Here's how the part is built. I have some questions about the finished solid (model axes, mm). Coordinates: 2 decimals unless noted, no trailing zeros. Write each loop counter-clockwise with the first axis right and the second up, starting at its lowest first coordinate (ties: lowest second). Pieces come first, ordered by that corner, then holes.
(1) Please list where these lines run through material, in increasing order: probe 1 along Y at (x, z) = (-4.5, 50); probe 2 along Z at (x, y) = (0, 70) (3 decimals); probe 3 along Z at (x, y) = (0, -1) (3 decimals).
(2) For pin 1 Ø1.5 at (x, y) = (11, 23.5) entering from +Z; pin 2 Ø2 at (x, y) = (16, -0.5) entering from +Z, each with a flat end and sliding along its axis, tell me the tip position at first contact or that it passes through.
(3) Thinking about a two-plate mould opening in Y: for faces 1 (the cylindrical face through (14.65, -1.07, -28.17)), 2 (the flat face through (0, -76.2, 37)), 3 (the flat face through (31.75, 64, 36)), which applies, released by +Y, released by -Y, zero draft, split by the parting line, or undercut?
(4) Imagine slicing it at D-D, the plane z = 75.5. List the corners of the cut face in (x, y) for me.
(5) Imagine slicing it at A-A, the plane z = 43. List the corners of the cut face in (x, y) for me.
(6) Imagine slicing it at C-C, the plane y = -54.5. List the corners of the cut face in (x, z) for me (3 decimals).
(7) Imagine slicing it at B-B, the plane x = 0. List the corners of the cut face in (y, z) for me (3 decimals).
```python
from build123d import *

# Parameters (mm, degrees)
F0_R     = 31.75
F0_R_2   = 15.875
F1_DEPTH = 76.2
F3_DEPTH = 25.4
F5_R     = 15.875
F6_DEPTH = 152.401


with BuildPart() as f1:
    # F0 (on Front) → F1 (new body, symmetric)
    with BuildSketch(Plane.XZ):
        Circle(F0_R)
        Circle(F0_R_2, mode=Mode.SUBTRACT)
    extrude(amount=F1_DEPTH, both=True)

    # F2 (on face) → F3 (join)
    with BuildSketch(Plane.XZ.offset(76.2)):
        with BuildLine():
            ThreePointArc((31.75, 72.5937485695), (0, 104.3437485695), (-31.75, 72.5937485695))
            Line((-31.75, 72.5937485695), (31.75, 72.5937485695))
        make_face()
        with BuildLine():
            Line((31.75, 72.5937485695), (-31.75, 72.5937485695))
            ThreePointArc((-31.75, 72.5937485695), (0, 40.8437485695), (31.75, 72.5937485695))
        make_face()
        with BuildLine():
            Line((-31.75, 72.5937485695), (-31.75, 0))
            ThreePointArc((-31.75, 0), (0, 31.75), (31.75, 0))
            Line((31.75, 0), (31.75, 72.5937485695))
            ThreePointArc((31.75, 72.5937485695), (0, 40.8437485695), (-31.75, 72.5937485695))
        make_face()
    extrude(amount=-F3_DEPTH)

    # F4: F1 across plane


with BuildPart() as f1_1:
    add(f1.part)
    add(f1.part.mirror(Plane.XZ))

    # F5 (on face) → F6 (cut, through all)
    with BuildSketch(Plane.XZ.offset(76.2)):
        with Locations((0, 72.5937485695)):
            Circle(F5_R)
    extrude(amount=-F6_DEPTH, mode=Mode.SUBTRACT)


solid = f1_1.part
```
Recorded:
1. probe 1: y = -76.2 to -50.8, 50.8 to 76.2
1. probe 2: z = -31.75 to -15.875, 15.875 to 56.719, 88.469 to 104.344
1. probe 3: z = -31.75 to -15.875, 15.875 to 31.75
2. pin 1: stops at z = 30.05
2. pin 2: stops at z = 27.98
3. face 1: undercut
3. face 2: released by -Y
3. face 3: zero draft
4. outline: (-31.62, -76.2) - (-15.61, -76.2) - (-15.61, -50.8) - (-31.62, -50.8) - close; (-31.62, 50.8) - (-15.61, 50.8) - (-15.61, 76.2) - (-31.62, 76.2) - close; (15.61, -76.2) - (31.62, -76.2) - (31.62, -50.8) - (15.61, -50.8) - close; (15.61, 50.8) - (31.62, 50.8) - (31.62, 76.2) - (15.61, 76.2) - close
5. outline: (-31.75, -76.2) - (31.75, -76.2) - (31.75, -50.8) - (-31.75, -50.8) - close; (-31.75, 50.8) - (31.75, 50.8) - (31.75, 76.2) - (-31.75, 76.2) - close
6. outline: (-31.75, 0) arc R31.75 ccw to (31.75, 0) - (31.75, 72.594) arc R31.75 ccw to (-31.75, 72.594) - close; hole circle Ø31.75 at (0, 0); hole circle Ø31.75 at (0, 72.594)
7. outline: (-76.2, -31.75) - (76.2, -31.75) - (76.2, -15.875) - (-76.2, -15.875) - close; (-76.2, 15.875) - (76.2, 15.875) - (76.2, 56.719) - (50.8, 56.719) - (50.8, 31.75) - (-50.8, 31.75) - (-50.8, 56.719) - (-76.2, 56.719) - close; (-76.2, 88.469) - (-50.8, 88.469) - (-50.8, 104.344) - (-76.2, 104.344) - close; (50.8, 88.469) - (76.2, 88.469) - (76.2, 104.344) - (50.8, 104.344) - close
